```python
from build123d import *

# Parameters (mm, degrees)
F2_DEPTH = 160


with BuildPart() as f2:
    # F1 (on Right) → F2 (new body, symmetric)
    with BuildSketch(Plane.YZ):
        with BuildLine():
            Line((19.709609, -22.585842), (-3.483844, -28.36862))
            ThreePointArc((-3.483844, -28.36862), (-4.576022, -29.077888), (-5, -30.309211))
            Line((-5, -30.309211), (-5, -45.5))
            ThreePointArc((-5, -45.5), (-4.414214, -46.914214), (-3, -47.5))
            Line((-3, -47.5), (0, -47.5))
            Line((0, -47.5), (0, -37.5))
            Line((0, -37.5), (30, -37.5))
            Line((30, -37.5), (30, -8.184728))
            ThreePointArc((30, -8.184728), (29.414693, -7.274767), (28.343941, -7.430018))
            Line((28.343941, -7.430018), (25.219705, -10.145875))
            ThreePointArc((25.219705, -10.145875), (23.950194, -11.845957), (23.5, -13.919423))
            Line((23.5, -13.919423), (23.5, -17.734364))
            ThreePointArc((23.5, -17.734364), (22.440054, -20.812671), (19.709609, -22.585842))
        make_face()
    extrude(amount=F2_DEPTH, both=True)


solid = f2.part
```
Here's how the part is built. I have some questions about the finished solid (model axes, mm). A direction names the side the tool comes from. Coordinates: 2 decimals unless noted, no trailing zeros. Loops run counter-clockwise (first coordinate to the right, second up) from the corner with the lowest first, then second, coordinate; pieces in that order, holes last. Notation, with made-up numbers: (76, 41.5) - (134, 41.5) arc R33 ccw to (134, 78.5) - close; hole circle Ø1 at (85, 36). An arc over 180 degrees is marked (long way). Answer as CSV lines item,"result".
Q1. For pin 1 (15 mm diameter, centred on x = -52, y = 11.5, fed in from -Z); pin 2 (1.1 mm diameter, centred on x = -79.5, z = -15, fed in from -Y); pin 3 (1.5 mm diameter, centred on x = -82.5, y = 4.5, fed in from +Z); pin 4 (4 mm diameter, centred on x = 40.5, z = -28.5, fed in from -Y), each with a flat end and sliding along its axis, tell me the tip position at first contact or that it passes through.
Response:
pin 1,"z = -37.5"
pin 2,"y = 23.5"
pin 3,"z = -26.19"
pin 4,"y = -5"
Q2. If we section it at B-B, the plane y = 5.5: Write out the boundary of the cut face in (x, z), and give its area (3 significant figures).
Response:
outline,"(-160, -37.5) - (160, -37.5) - (160, -26.13) - (-160, -26.13) - close"
area,"3,640 mm2"
Q3. If we section it at C-C, the plane y = 17: Write out the boundary of the cut face in (x, z).
Response:
outline,"(-160, -37.5) - (160, -37.5) - (160, -23.26) - (-160, -23.26) - close"
Q4. If I drill on L1, parallel to Y at x = -84.5, z = -44.5; L2, parallel to Z at x = 114.5, y = 2; L3, parallel to Z at x = -50, y = 11.5, over which ranges is the centre line in solid material (lowest first)? Write a range as [from, to].
Response:
L1,"[-5, 0]"
L2,"[-37.5, -27]"
L3,"[-37.5, -24.63]"
Q5. If we section it at A-A, the plane x = 111.5: Write out the boundary of the cut face in (y, z).
Response:
outline,"(-5, -45.5) arc R2 ccw to (-3, -47.5) - (0, -47.5) - (0, -37.5) - (30, -37.5) - (30, -8.18) arc R1 ccw to (28.34, -7.43) - (25.22, -10.15) arc R5 ccw to (23.5, -13.92) - (23.5, -17.73) arc R5 cw to (19.71, -22.59) - (-3.48, -28.37) arc R2 ccw to (-5, -30.31) - close"
Q6. For faces 1 (the face through (2, 15, -37.5)), 2 (the face through (2, -5, -38)), which set-ups out of +Z, -Z, +X, -X, +Y, -Y let a thin tool reach every point of the face, with its end or its side?
Response:
face 1,"-Z, +X, -X, +Y"
face 2,"+Z, -Z, +X, -X, -Y"
